Part model, mm, in its own coordinate system. A direction names the side the tool comes from. Coordinates: 2 decimals unless noted, no trailing zeros. Loops run counter-clockwise (first coordinate to the right, second up) from the corner with the lowest first, then second, coordinate; pieces in that order, holes last. Notation, with made-up numbers: (41, 83.5) -> (61, 83.5) arc R33 cw to (61, 114.5) -> close; hole circle Ø8 at (-23.5, -7). An arc over 180 degrees is marked (long way). Use one line per item in the form item = value. Start each with the question number.
(1) Band-saw the part on B-B on y = 476. Give the cut face in (x, z).
(2) Pin check, flat tip, straight feed: P1, Ø1.5, axis at x = 534, y = 222, coming from the -Z side. Stop position of the tip, or through.
(3) 3-axis set-ups, long thin cutter, end or side, ignore diameter. For faces 1 (the flat face through (500, 50, 139)), 2 (the flat face through (465, 247, 163)), 3 (the flat face through (965, 377, 165)), 4 (the flat face through (965, 127, 280)), 5 (the flat face through (728, 680, 25)): which of +Z, -Z, +X, -X, +Y, -Y reach the whole face in a straight line?
(4) Band-saw the part on A-A on z = 197.5. Give the cut face in (x, y), then the cut area to 3 significant figures.
(5) Band-saw the part on D-D on z = 248.5. Give the cut face in (x, y), then the cut area to 3 significant figures.
(6) Band-saw the part on C-C on x = 322.5. Give the cut face in (y, z), then the cut area to 3 significant figures.
(7) Drill centre lines: L1, parallel to X at y = 326.5, z = 12.5; L2, parallel to Y at x = 526, z = 226; L3, parallel to X at y = 32.5, z = 257. Where is each one in solid material? Low to high. Write a range as [from, to].
(8) Mould opens along Z. For faces 6 (the flat face through (35, 377, 165)), 7 (the flat face through (263, 70, 25)), 8 (the flat face through (500, 250, 82)) say: +Z half, -Z half, draft (parallel to the pull), parting line (faces both ways), or undercut.
```python
from build123d import *

# Parameters (mm, degrees)
SKETCH_W                   = 1000
SKETCH_H                   = 750
SKETCH_W_2                 = 392.088353
SKETCH_H_2                 = 610
SKETCH_W_3                 = 397.911647
PAD_DEPTH                  = 50
SKETCH001_W                = 70
SKETCH001_H                = 50
PAD001_DEPTH               = 180
SKETCH001_MIRRORED001_2_W  = 70
SKETCH001_MIRRORED001_2_H  = 50
PAD001_MIRRORED001_2_DEPTH = 180
LINEARPATTERN_COUNT        = 3
LINEARPATTERN_PITCH        = 465
SKETCH002_W                = 70
SKETCH002_H                = 50
PAD002_DEPTH               = 65
SKETCH003_W                = 70
SKETCH003_H                = 250
PAD003_DEPTH               = 50
LINEARPATTERN001_COUNT     = 3
LINEARPATTERN001_PITCH     = 465
LINEARPATTERN002_COUNT     = 3
LINEARPATTERN002_PITCH     = 465
SKETCH004_W                = 70
SKETCH004_H                = 250
PAD004_DEPTH               = 50
LINEARPATTERN003_COUNT     = 3
LINEARPATTERN003_PITCH     = 465


with BuildPart() as part:
    # Sketch → Pad (new body)
    with BuildSketch(Plane.XY):
        with Locations((500, 375)):
            Rectangle(SKETCH_W, SKETCH_H)
        with Locations((266.044176, 375)):
            Rectangle(SKETCH_W_2, SKETCH_H_2, mode=Mode.SUBTRACT)
        with Locations((731.044177, 375)):
            Rectangle(SKETCH_W_3, SKETCH_H_2, mode=Mode.SUBTRACT)
    extrude(amount=PAD_DEPTH)

    # Sketch001 → Pad001 (join)
    with BuildSketch(Plane.XY.offset(50)):
        with Locations((35, 25)):
            Rectangle(SKETCH001_W, SKETCH001_H)
    pad001 = extrude(amount=PAD001_DEPTH)

    # Sketch001 Mirrored001 2 → Pad001 Mirrored001 2 (add)
    with BuildSketch(Plane(origin=(0, 250, 50), x_dir=(1, 0, 0), z_dir=(0, 0, -1))):
        with Locations((35, 25)):
            Rectangle(SKETCH001_MIRRORED001_2_W, SKETCH001_MIRRORED001_2_H)
    pad001_mirrored001_2 = extrude(amount=-PAD001_MIRRORED001_2_DEPTH)

    # LinearPattern: Pad001, Pad001 Mirrored001 2 ×3
    with Locations(*[(i * LINEARPATTERN_PITCH, 0, 0) for i in range(1, LINEARPATTERN_COUNT)]):
        add(pad001)
        add(pad001_mirrored001_2)

    # Sketch002 → Pad002 (join)
    with BuildSketch(Plane.XY.offset(50)):
        with Locations((35, 475)):
            Rectangle(SKETCH002_W, SKETCH002_H)
    pad002 = extrude(amount=PAD002_DEPTH)

    # Sketch003 (on DatumPlane) → Pad003 (join)
    with BuildSketch(Plane.XY.offset(230)):
        with Locations((35, 125)):
            Rectangle(SKETCH003_W, SKETCH003_H)
    pad003 = extrude(amount=PAD003_DEPTH)

    # LinearPattern001: Pad002 ×3
    with Locations(*[(i * LINEARPATTERN001_PITCH, 0, 0) for i in range(1, LINEARPATTERN001_COUNT)]):
        add(pad002)

    # LinearPattern002: Pad003 ×3
    with Locations(*[(i * LINEARPATTERN002_PITCH, 0, 0) for i in range(1, LINEARPATTERN002_COUNT)]):
        add(pad003)

    # Sketch004 (on DatumPlane) → Pad004 (join)
    with BuildSketch(Plane.XY.offset(115)):
        with Locations((35, 375)):
            Rectangle(SKETCH004_W, SKETCH004_H)
    pad004 = extrude(amount=PAD004_DEPTH)

    # LinearPattern003: Pad004 ×3
    with Locations(*[(i * LINEARPATTERN003_PITCH, 0, 0) for i in range(1, LINEARPATTERN003_COUNT)]):
        add(pad004)


solid = part.part
```
A:
q1.outline = (0, 0) -> (70, 0) -> (70, 165) -> (0, 165) -> close; (462.09, 0) -> (532.09, 0) -> (532.09, 50) -> (535, 50) -> (535, 165) -> (465, 165) -> (465, 50) -> (462.09, 50) -> close; (930, 0) -> (1000, 0) -> (1000, 165) -> (930, 165) -> close
q2.P1 = 50
q3.face_1 = +X, -X
q3.face_2 = +Z, +Y, -Y
q3.face_3 = +Z, +X, -X, +Y
q3.face_4 = +Z, +X, -X, +Y, -Y
q3.face_5 = +Z, -Z
q4.outline = (0, 0) -> (70, 0) -> (70, 50) -> (0, 50) -> close; (0, 200) -> (70, 200) -> (70, 250) -> (0, 250) -> close; (465, 0) -> (535, 0) -> (535, 50) -> (465, 50) -> close; (465, 200) -> (535, 200) -> (535, 250) -> (465, 250) -> close; (930, 0) -> (1000, 0) -> (1000, 50) -> (930, 50) -> close; (930, 200) -> (1000, 200) -> (1000, 250) -> (930, 250) -> close
q4.area = 21,000 mm²
q5.outline = (0, 0) -> (70, 0) -> (70, 250) -> (0, 250) -> close; (465, 0) -> (535, 0) -> (535, 250) -> (465, 250) -> close; (930, 0) -> (1000, 0) -> (1000, 250) -> (930, 250) -> close
q5.area = 52,500 mm²
q6.outline = (0, 0) -> (70, 0) -> (70, 50) -> (0, 50) -> close; (680, 0) -> (750, 0) -> (750, 50) -> (680, 50) -> close
q6.area = 7,000 mm²
q7.L1 = [0, 70], [462.09, 532.09], [930, 1000]
q7.L2 = [0, 50], [200, 250]
q7.L3 = [0, 70], [465, 535], [930, 1000]
q8.face_6 = +Z half
q8.face_7 = draft
q8.face_8 = undercut
